Drawing for the job (mm, zero at the part's lowest x, y, z). A direction names the side the tool comes from. Give positions to 0.01 mm unless a question says otherwise; leave off trailing zeros. Write each loop counter-clockwise with the first axis right and the second up, starting at its lowest first coordinate (ties: lowest second). Pieces come first, ordered by that corner, then holes. Notation, with made-up numbers: (24.25, 68) - (34.25, 68) arc R13 cw to (34.25, 87) - close; hole circle Ø4 at (-24.75, 40.5). An arc over 180 degrees is marked (long way). Answer as a JSON object with one key per item and string values. Group by question number.
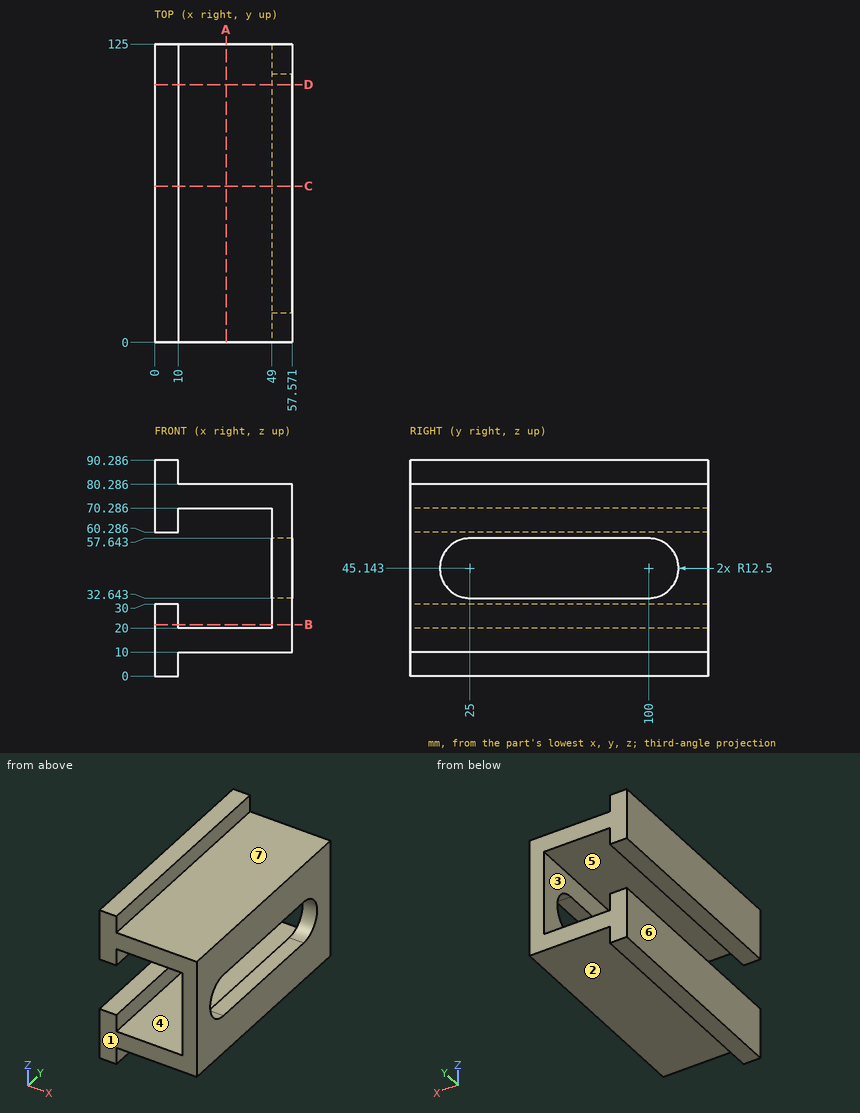
1) Band-saw the part on C-C (y = 65.5). List the corners of the cut face in (x, z) (1 decimal), plus the area to 3 significant figures.
2) Band-saw the part on A-A (x = 30). List the corners of the cut face in (y, z) (1 decimal), plus the area to 3 significant figures.
3) Band-saw the part on D-D (y = 108). List the corners of the cut face in (x, z) (1 decimal), plus the area to 3 significant figures.
4) Drop flat-ended pins along their axis: P1, Ø3, axis at x = 41, y = 35, coming from the +Z side; P2, Ø2.5, axis at x = 53, y = 77, coming from the -Z side; P3, Ø25, axis at y = 87, z = 45, coming from the -X side. Give the stop position or say it passes through.
5) Probe line 1 (Z direction, x = 46, y = 90.5) (1 decimal); line 2 (Z direction, x = 4.5, y = 40) (1 decimal); line 3 (X direction, y = 99.5, z = 32). List the from-to ranges inside material, lowest first.
6) Mould opens along Z. For the marked faces 4, 5, 6 and 7 say: pulls with the +Z half, pulls with the -Z half, needs draft (parallel to the pull), parting line crosses it, or undercut.
7) Which spindle directions (+Z, -Z, +X, -X, +Y, -Y) get a long thin tool onto all of the face, cutting with end or side? Do the marked faces 1, 2 and 3. Say none if no direction does.
8) Band-saw the part on B-B (z = 21.5). List the corners of the cut face in (x, y), plus the area to 3 significant figures.
Verdict:
{
 "1": {"outline": "(0, 0) - (10, 0) - (10, 10) - (57.6, 10) - (57.6, 32.6) - (49, 32.6) - (49, 20) - (10, 20) - (10, 30) - (0, 30) - close; (0, 60.3) - (10, 60.3) - (10, 70.3) - (49, 70.3) - (49, 57.6) - (57.6, 57.6) - (57.6, 80.3) - (10, 80.3) - (10, 90.3) - (0, 90.3) - close", "area": "1,770 mm2"},
 "2": {"outline": "(0, 10) - (125, 10) - (125, 20) - (0, 20) - close; (0, 70.3) - (125, 70.3) - (125, 80.3) - (0, 80.3) - close", "area": "2,500 mm2"},
 "3": {"outline": "(0, 0) - (10, 0) - (10, 10) - (57.6, 10) - (57.6, 35.5) - (49, 35.5) - (49, 20) - (10, 20) - (10, 30) - (0, 30) - close; (0, 60.3) - (10, 60.3) - (10, 70.3) - (49, 70.3) - (49, 54.7) - (57.6, 54.7) - (57.6, 80.3) - (10, 80.3) - (10, 90.3) - (0, 90.3) - close", "area": "1,820 mm2"},
 "4": {"P1": "z = 80.29", "P2": "z = 10", "P3": "x = 49"},
 "5": {"line 1": "10 to 20, 70.3 to 80.3", "line 2": "0 to 30, 60.3 to 90.3", "line 3": "49 to 57.57"},
 "6": {"face 4": "undercut", "face 5": "undercut", "face 6": "needs draft", "face 7": "pulls with the +Z half"},
 "7": {"face 1": "+Z, -Z, +X, -X, -Y", "face 2": "-Z, +X, +Y, -Y", "face 3": "+Y, -Y"},
 "8": {"outline": "(0, 0) - (10, 0) - (10, 125) - (0, 125) - close; (49, 0) - (57.57, 0) - (57.57, 125) - (49, 125) - close", "area": "2,320 mm2"}
}
